For this review, take the finished solid that the model builds, in its own axes (mm). A direction names the side the tool comes from. Round coordinates to 2 decimals unless told otherwise and drop trailing zeros. Order: outer loops, then holes, each group sorted by start corner. A loop starts at its lowest first (then second) coordinate and runs counter-clockwise, first axis right, second up. Notation, with made-up numbers: M -18.75,-30.75 L 30.25,-30.75 A23 cw 30.25,-5.75 Z; hole C 78.5,88 d6. An arc over 180 degrees is marked long. Use a Markdown table: item, result.
from build123d import *

# Parameters (mm, degrees)
SKETCH1_W               = 150
SKETCH1_H               = 140
SKETCH1_W_2             = 130
SKETCH1_H_2             = 120
BOSS_EXTRUDE1_DEPTH     = 150
BOSS_EXTRUDE2_DEPTH     = 10
BOSS_EXTRUDE3_DEPTH     = 10
SKETCH7_W               = 130
SKETCH7_H               = 150
CUT_EXTRUDE2_DEPTH      = 140
SKETCH8_W               = 10
SKETCH8_H               = 140
BOSS_EXTRUDE4_DEPTH     = 150
CUT_EXTRUDE3_DEPTH      = 1
CUT_EXTRUDE3_DEPTH_BACK = 150


with BuildPart() as part:
    # Sketch1 → Boss-Extrude1 (new body)
    with BuildSketch(Plane.XY):
        Rectangle(SKETCH1_W, SKETCH1_H)
        Rectangle(SKETCH1_W_2, SKETCH1_H_2, mode=Mode.SUBTRACT)
    extrude(amount=BOSS_EXTRUDE1_DEPTH)

    # Sketch3 → Boss-Extrude2 (add)
    with BuildSketch(Plane(origin=(75, 0, 0), x_dir=(0, 0, -1), z_dir=(1, 0, 0))):
        with BuildLine():
            Line((30, 15), (0, 15))
            Line((0, 15), (0, -15))
            Line((0, -15), (30, -15))
            Line((30, -15), (30, -2.5))
            Line((30, -2.5), (22.071067812, -2.5))
            ThreePointArc((22.071067812, -2.5), (7.5, 0), (22.071067812, 2.5))
            Line((22.071067812, 2.5), (30, 2.5))
            Line((30, 2.5), (30, 15))
        make_face()
    extrude(amount=-BOSS_EXTRUDE2_DEPTH)

    # Sketch4 → Boss-Extrude3 (add)
    with BuildSketch(Plane.ZY.offset(75)):
        with BuildLine():
            Line((0, -15), (0, 15))
            Line((0, 15), (-30, 15))
            Line((-30, 15), (-30, 2.5))
            Line((-30, 2.5), (-22.071067812, 2.5))
            ThreePointArc((-22.071067812, 2.5), (-13.73173516, 7.391989197), (-7.5, 0))
            ThreePointArc((-7.5, 0), (-13.73173516, -7.391989197), (-22.071067812, -2.5))
            Line((-22.071067812, -2.5), (-30, -2.5))
            Line((-30, -2.5), (-30, -15))
            Line((-30, -15), (0, -15))
        make_face()
    extrude(amount=-BOSS_EXTRUDE3_DEPTH)

    # Sketch7 → Cut-Extrude2 (cut)
    with BuildSketch(Plane.XZ.offset(70)):
        with Locations((0, 75)):
            Rectangle(SKETCH7_W, SKETCH7_H)
    extrude(amount=-CUT_EXTRUDE2_DEPTH, mode=Mode.SUBTRACT)

    # Sketch8 → Boss-Extrude4 (add)
    with BuildSketch(Plane.ZY.offset(75)):
        with Locations((145, 0)):
            Rectangle(SKETCH8_W, SKETCH8_H)
    extrude(amount=-BOSS_EXTRUDE4_DEPTH)

    # Sketch9 → Cut-Extrude3 (cut, two sides)
    with BuildSketch(Plane.ZY.offset(75)) as cut_extrude3_sk:
        Polygon((0, -15), (140, -70), (0, -70), align=None)
        Polygon((0, 15), (0, 70), (140, 70), align=None)
    extrude(amount=CUT_EXTRUDE3_DEPTH, mode=Mode.SUBTRACT)
    extrude(cut_extrude3_sk.sketch, amount=-CUT_EXTRUDE3_DEPTH_BACK, mode=Mode.SUBTRACT)


solid = part.part
Q1. Machinability: for faces 1 (the flat face through (65, -1, 73)), 2 (the flat face through (-70, 15, -15)), 3 (the flat face through (-70, -2.5, -26)), which of the approach directions +Z, -Z, +X, -X, +Y, -Y give a long, thin tool a straight path to every point of the face, cutting with its end or side? Answer none if there is none.
Determined:
| item | result |
|---|---|
| face 1 | -Z, +Y, -Y |
| face 2 | -Z, +X, -X, +Y |
| face 3 | -Z, +X, -X |
Q2. Add section A-A (z = -15). Write out the cut boundary in (x, y).
Determined:
| item | result |
|---|---|
| outline | M -75,-15 L -65,-15 L -65,-7.5 L -75,-7.5 Z; M -75,7.5 L -65,7.5 L -65,15 L -75,15 Z; M 65,-15 L 75,-15 L 75,-7.5 L 65,-7.5 Z; M 65,7.5 L 75,7.5 L 75,15 L 65,15 Z |
Q3. Add section D-D (z = 108). Write out the cut boundary in (x, y).
Determined:
| item | result |
|---|---|
| outline | M -75,-57.43 L -65,-57.43 L -65,57.43 L -75,57.43 Z; M 65,-57.43 L 75,-57.43 L 75,57.43 L 65,57.43 Z |
Q4. Add section B-B (z = 39.5). Write out the cut boundary in (x, y).
Determined:
| item | result |
|---|---|
| outline | M -75,-30.52 L -65,-30.52 L -65,30.52 L -75,30.52 Z; M 65,-30.52 L 75,-30.52 L 75,30.52 L 65,30.52 Z |
Q5. Draft analysis for pull direction Y (two halves, no side actions). For faces 4 (the flat face through (70, 9, -30)), 5 (the flat face through (69.93, 42.885, 70.98)), 6 (the flat face through (70, 2.5, -26)), state which applies: pulls with the +Y half, pulls with the -Y half, needs draft (parallel to the pull), parting line crosses it, or undercut.
Determined:
| item | result |
|---|---|
| face 4 | needs draft |
| face 5 | pulls with the +Y half |
| face 6 | undercut |
Q6. Add section C-C (y = -30.5). Write out the cut boundary in (x, z).
Determined:
| item | result |
|---|---|
| outline | M -75,39.45 L -65,39.45 L -65,140 L 65,140 L 65,39.45 L 75,39.45 L 75,150 L -75,150 Z |
Q7. Wall thickness on line 1 along Y through (x, z) = (70, -15); line 2 along X through (y, z) = (45.5, 104.5); line 3 along Z through (x, y) = (-17, -29): over which ranges is each line inside the solid? List them lowest first. Write a range as [from, to].
Determined:
| item | result |
|---|---|
| line 1 | y = [-15, -7.5], [7.5, 15] |
| line 2 | x = [-75, -65], [65, 75] |
| line 3 | z = [140, 150] |
Q8. Clearance check with flat-ended pins moving along their axes: pin 1 (6.5 mm diameter, centred on x = 72.5, z = -26, fed in from +Y); pin 2 (24 mm diameter, centred on y = 0, z = -15, fed in from -X); pin 3 (4 mm diameter, centred on x = 68, z = -26, fed in from -Y). State where each tip first meets the part, or that it passes through.
Determined:
| item | result |
|---|---|
| pin 1 | stops at y = 15 |
| pin 2 | stops at x = -75 |
| pin 3 | stops at y = -15 |
